Design review of the part built by this model. Coordinates are the model's own, in mm. Face numbers are marked on the shaded views. Coordinates: 2 decimals unless noted, no trailing zeros. Write each loop counter-clockwise with the first axis right and the second up, starting at its lowest first coordinate (ties: lowest second). Pieces come first, ordered by that corner, then holes. Notation, with made-up numbers: (-26, 22) -> (-14, 22) arc R21 ccw to (-14, 54) -> close; hole circle Ø4 at (-23.75, 8.25). An arc over 180 degrees is marked (long way). Write item = value, one per line. Start each with the question number.
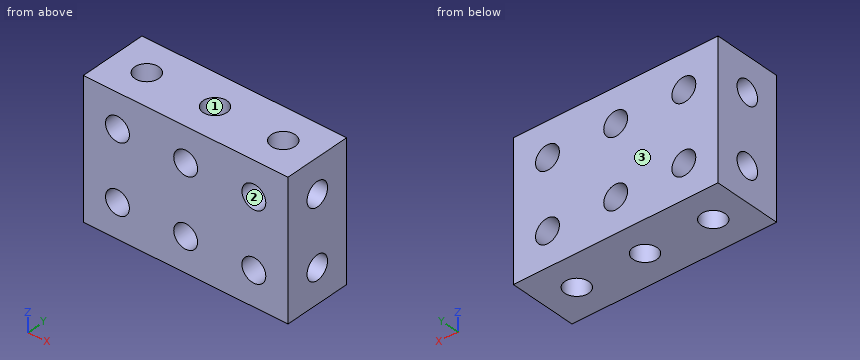
```python
from build123d import *

# Parameters (mm, degrees)
ESQUISSE1_W             = 20
ESQUISSE1_H             = 10
BOSS_EXTRU_1_DEPTH      = 30
ESQUISSE2_R             = 1.75
ENL_V_MAT_EXTRU_1_DEPTH = 38.416573868
ESQUISSE3_R             = 1.75
ENL_V_MAT_EXTRU_2_DEPTH = 40
ESQUISSE4_R             = 1.75
ENL_V_MAT_EXTRU_3_DEPTH = 40


with BuildPart() as part:
    # Esquisse1 → Boss.-Extru.1 (new body)
    with BuildSketch(Plane(origin=(0, 0, 0), x_dir=(0, 0, -1), z_dir=(1, 0, 0))):
        with Locations((10, 5)):
            Rectangle(ESQUISSE1_W, ESQUISSE1_H)
    extrude(amount=BOSS_EXTRU_1_DEPTH)

    # Esquisse2 → Enlèv. mat.-Extru.1 (cut, through all)
    with BuildSketch(Plane(origin=(0, 10, 0), x_dir=(1, 0, 0), z_dir=(0, 1, 0))):
        with Locations(Location((5, 15, 0), (0, 0, 270))):
            Circle(ESQUISSE2_R)
        with Locations(Location((15, 15, 0), (0, 0, 270))):
            Circle(ESQUISSE2_R)
        with Locations(Location((25, 15, 0), (0, 0, 270))):
            Circle(ESQUISSE2_R)
        with Locations((35, 15)):
            Circle(ESQUISSE2_R)
        with Locations(Location((5, 5, 0), (0, 0, 270))):
            Circle(ESQUISSE2_R)
        with Locations(Location((15, 5, 0), (0, 0, 270))):
            Circle(ESQUISSE2_R)
        with Locations(Location((25, 5, 0), (0, 0, 270))):
            Circle(ESQUISSE2_R)
        with Locations((35, 5)):
            Circle(ESQUISSE2_R)
        with Locations((5, -5)):
            Circle(ESQUISSE2_R)
        with Locations((15, -5)):
            Circle(ESQUISSE2_R)
        with Locations((25, -5)):
            Circle(ESQUISSE2_R)
        with Locations((35, -5)):
            Circle(ESQUISSE2_R)
        with Locations((5, -15)):
            Circle(ESQUISSE2_R)
        with Locations((15, -15)):
            Circle(ESQUISSE2_R)
        with Locations((25, -15)):
            Circle(ESQUISSE2_R)
        with Locations((35, -15)):
            Circle(ESQUISSE2_R)
    extrude(amount=-ENL_V_MAT_EXTRU_1_DEPTH, mode=Mode.SUBTRACT)

    # Esquisse3 → Enlèv. mat.-Extru.2 (cut)
    with BuildSketch(Plane.XY):
        with Locations((5, 5)):
            Circle(ESQUISSE3_R)
        with Locations((15, 5)):
            Circle(ESQUISSE3_R)
        with Locations((25, 5)):
            Circle(ESQUISSE3_R)
        with Locations((35, 5)):
            Circle(ESQUISSE3_R)
    extrude(amount=-ENL_V_MAT_EXTRU_2_DEPTH, mode=Mode.SUBTRACT)

    # Esquisse4 → Enlèv. mat.-Extru.3 (cut)
    with BuildSketch(Plane(origin=(30, 0, 0), x_dir=(0, 0, -1), z_dir=(1, 0, 0))):
        with Locations((5, 5)):
            Circle(ESQUISSE4_R)
        with Locations(Location((15, 5, 0), (0, 0, 315))):
            Circle(ESQUISSE4_R)
        with Locations((25, 5)):
            Circle(ESQUISSE4_R)
        with Locations((35, 5)):
            Circle(ESQUISSE4_R)
    extrude(amount=-ENL_V_MAT_EXTRU_3_DEPTH, mode=Mode.SUBTRACT)


solid = part.part
```
(1) Take a section at C-C, the plane z = -18. State the section outline as (x, y) points, then the cut area to 3 significant figures.
(2) Take a section at B-B, the plane y = 9. State the section outline as (x, z) points.
(3) For pin 1 Ø3 at (x, y) = (25, 5) entering from -Z, flat-tipped, find the tip position at first contact; note if it passes through.
(4) Take a section at D-D, the plane x = 14.5. State the section outline as (y, z) points, then the cut area to 3 significant figures.
(5) For line 1 (X direction, y = 1.25, z = -15); line 2 (Z direction, x = 25, y = 9.2); line 3 (Y direction, x = 20, z = -15), list the stretches that pass through material, from the lowest coordinate up.
(6) Take a section at A-A, the plane z = -15. Count the separate pieces of the cut face and the enclosed holes in it, then the cut area to 3 significant figures.
(7) Mouldability with a two-part tool opening along Y and no side actions: class the marked faces 1, 2 and 3 as pulls with the +Y half, pulls with the -Y half, needs draft (parallel to the pull), parting line crosses it, or undercut.
Report:
q1.outline = (0, 0) -> (30, 0) -> (30, 10) -> (0, 10) -> close; hole circle Ø3.5 at (5, 5); hole circle Ø3.5 at (15, 5); hole circle Ø3.5 at (25, 5)
q1.area = 271 mm2
q2.outline = (0, -20) -> (30, -20) -> (30, 0) -> (0, 0) -> close; hole circle Ø3.5 at (5, -15); hole circle Ø3.5 at (5, -5); hole circle Ø3.5 at (15, -15); hole circle Ø3.5 at (15, -5); hole circle Ø3.5 at (25, -15); hole circle Ø3.5 at (25, -5)
q3.pin_1 = through
q4.outline = (0, -20) -> (3.32, -20) -> (3.32, -16.68) -> (0, -16.68) -> close; (0, -13.32) -> (3.32, -13.32) -> (3.32, -6.68) -> (0, -6.68) -> close; (0, -3.32) -> (3.32, -3.32) -> (3.32, 0) -> (0, 0) -> close; (6.68, -20) -> (10, -20) -> (10, -16.68) -> (6.68, -16.68) -> close; (6.68, -13.32) -> (10, -13.32) -> (10, -6.68) -> (6.68, -6.68) -> close; (6.68, -3.32) -> (10, -3.32) -> (10, 0) -> (6.68, 0) -> close
q4.area = 88.3 mm2
q5.line_1 = 0 to 3.25, 6.75 to 13.25, 16.75 to 23.25, 26.75 to 30
q5.line_2 = -20 to -16.75, -13.25 to -6.75, -3.25 to 0
q5.line_3 = 0 to 3.25, 6.75 to 10
q6.separate_pieces = 8
q6.enclosed_holes = 0
q6.area = 127 mm2
q7.face_1 = undercut
q7.face_2 = needs draft
q7.face_3 = pulls with the +Y half
